Autodesk Fusion 360 part; units mm, degrees
sketch "polarizer frame" plane through (0, 0, 0) normal (0, 0, 1) x (1, 0, 0)
  line L0 (130, 48) -> (130, -54)
  line L1 (130, -54) -> (232, -54)
  line L2 (234, 63) -> (247, 63)
  line L3 (247, -54) -> (247, -67)
  line L4 (117, 63) -> (117, 58)
  circle A0 centre (122, 58) radius 2
  line L5 (247, 63) -> (247, 58)
  circle A1 centre (242, 58) radius 2
  line L6 (247, -67) -> (242, -67)
  circle A2 centre (242, -62) radius 2
  line L7 (117, -67) -> (122, -67)
  circle A3 centre (122, -62) radius 2
  circle A4 centre (236.3431, 52.3431) radius 2
  line L8 (232, 48) -> (232, -54)
  line L9 (232, 48) -> (130, 48)
  line L10 (135, 63) -> (135, 59)
  line L11 (247, 63) -> (229, 63)
  line L12 (229, 63) -> (229, 59)
  line L13 (135, 59) -> (135, 57)
  line L14 (135, 57) -> (229, 56)
  line L15 (229, 56) -> (229, 59)
  line L16 (117, 63) -> (135, 63)
  line L17 (229, 63) -> (247, 63)
  line L18 (117, 63) -> (117, 45)
  line L19 (117, 45) -> (123, 45)
  line L20 (117, -67) -> (117, -49)
  line L21 (117, -49) -> (123, -49)
  line L22 (123, -49) -> (123, 45)
  line L23 (117, -67) -> (117, -49)
  line L24 (117, 45) -> (117, 63)
  line L25 (247, 63) -> (247, 45)
  line L26 (247, -67) -> (247, -49)
  line L27 (247, -49) -> (241, -49)
  line L28 (247, 45) -> (241, 45)
  line L29 (241, 45) -> (241, -49)
  line L30 (247, 63) -> (247, 45)
  line L31 (247, -49) -> (247, -54)
  line L32 (117, -67) -> (135, -67)
  line L33 (247, -67) -> (229, -67)
  line L34 (135, -67) -> (135, -61)
  line L35 (135, -61) -> (229, -61)
  line L36 (229, -61) -> (229, -67)
  line L37 (247, -67) -> (229, -67)
  line L38 (135, -67) -> (117, -67)
  dimension "d21" = 13
  dimension "d22" = 13
  dimension "d23" = 130
  dimension "d24" = 130
  dimension "d25" = 5
  dimension "d26" = 4
  dimension "d27" = 5
  dimension "d28" = 5
  dimension "d29" = 4
  dimension "d30" = 4
  dimension "d31" = 4
  dimension "d43" = 8
  dimension "d44" = 4
  dimension "d47" = 18
  dimension "d48" = 4
  dimension "d49" = 18
  dimension "d50" = 18
  dimension "d51" = 6
  dimension "d52" = 18
  dimension "d53" = 18
  dimension "d54" = 6
  dimension "d55" = 6
  dimension "d56" = 18
  dimension "d57" = 18
  dimension "d58" = 6
extrude "Extrude7" add sketch "polarizer frame" along normal blind 2.25
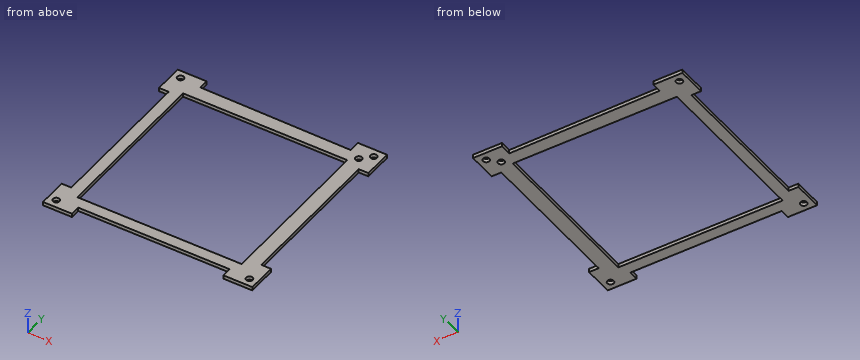
CAD build for the part. Positions are in the model's coordinates, mm. Round coordinates to 2 decimals unless told otherwise and drop trailing zeros. Loops run counter-clockwise (first coordinate to the right, second up) from the corner with the lowest first, then second, coordinate; pieces in that order, holes last. Notation, with made-up numbers: M 68.25,-25 L 115.25,-25 A6 cw 115.25,-14 Z; hole C 61,46.25 d5. An arc over 180 degrees is marked long. Return JSON: item names as keys, results as strings. Group by question number.
(1) Saw through at C-C, the plane z = 0.6. Give the number of separate pieces and of enclosed holes in the cut face, and give its area (3 significant figures).
(2) Wall check: probe 1 along Y at (x, z) = (122, 1.7); probe 2 along X at (y, z) = (-23, 2.1); probe 3 along Y at (x, z) = (231.5, 1.55). Give the ranges that are in metal, low to high. Write a range as [from, to].
(3) Saw through at A-A, the plane y = 1.5. List the corners of the cut face in (x, z), and give its area (3 significant figures).
(4) Drop flat-ended pins along their axis: P1, Ø1.1, axis at y = -21.5, z = 1.5, coming from the +X side; P2, Ø3, axis at x = 236.34, y = 52.34, coming from the -Z side; P3, Ø1.1, axis at x = 191, z = 1, coming from the -Y side. Give the stop position or say it passes through.
(5) Saw through at B-B, the plane x = 215. List the corners of the cut face in (y, z).
Answer list:
{
 "1": {"separate pieces": "1", "enclosed holes": "6", "area": "4,130 mm2"},
 "2": {"probe 1": "[-67, -64], [-60, -49], [45, 56], [60, 63]", "probe 2": "[123, 130], [232, 241]", "probe 3": "[-67, -54], [48, 63]"},
 "3": {"outline": "M 123,0 L 130,0 L 130,2.25 L 123,2.25 Z; M 232,0 L 241,0 L 241,2.25 L 232,2.25 Z", "area": "36.0 mm2"},
 "4": {"P1": "x = 241", "P2": "through", "P3": "y = -61"},
 "5": {"outline": "M -61,0 L -54,0 L -54,2.25 L -61,2.25 Z; M 48,0 L 56.15,0 L 56.15,2.25 L 48,2.25 Z"}
}
